```python
from build123d import *

# Parameters (mm, degrees)
EXTRUDE_1_DEPTH   = 2
HOLE_WIZARD_M81_D = 9
CHAMFER_1_SIZE    = 2


with BuildPart() as part:
    # Эскиз1 → Бобышка-Вытянуть1 (new body)
    with BuildSketch(Plane(origin=(0, 0, 0), x_dir=(1, 0, 0), z_dir=(0, 0, -1))):
        Polygon((0, 0), (0, 100), (100, 100), (100, 50), (50, 0), align=None)
    extrude(amount=EXTRUDE_1_DEPTH)

    # Отверстие с зазором M81 (through all)
    with Locations(Plane(origin=(0, 0, -2), x_dir=(1, 0, 0), z_dir=(0, 0, -1))):
        with Locations((25, 75), (25, 25), (75, 75)):
            Hole(HOLE_WIZARD_M81_D / 2)

    # Фаска1
    chamfer_1_edges = [part.edges().sort_by_distance(p)[0] for p in [
        (0, 0, -1),
        (0, -100, -1),
        (100, -100, -1),
    ]]
    chamfer(chamfer_1_edges, length=CHAMFER_1_SIZE)


solid = part.part
```
CAD build for the part. Positions are in the model's coordinates, mm. Round coordinates to 2 decimals unless told otherwise and drop trailing zeros. Order: outer loops, then holes, each group sorted by start corner. A loop starts at its lowest first (then second) coordinate and runs counter-clockwise, first axis right, second up. Notation, with made-up numbers: (-3, 82) - (45, 82) arc R9 ccw to (45, 95) - close; hole circle Ø10 at (33, 20.5). An arc over 180 degrees is marked (long way). Use CSV: the item, a comma, the result in double quotes. Start each with the question number.
1) Saw through at A-A (y = -75). List the corners of the cut face in (x, z).
2) Saw through at D-D (z = -1.2). List the corners of the cut face in (x, y), and give its area (3 significant figures).
3) Wall check: L1, parallel to X at y = -75, z = -0.6; L2, parallel to Y at x = 26, z = -1.35; L3, parallel to Y at x = 75, z = -0.5. Give the ranges that are in metal, low to high. Write a range as [from, to].
4) Saw through at B-B (x = 75). List the corners of the cut face in (y, z), and give its area (3 significant figures).
5) Saw through at C-C (y = -25). List the corners of the cut face in (x, z), and give its area (3 significant figures).
6) Two-plate mould, pull along X, no slides. Class faces 1 (the flat face through (51, -51, 0)), 2 (the flat face through (75, -25, -1)), 3 (the cylindrical face through (28.32, -28.04, -0.99)): pulls with the +X half, pulls with the -X half, needs draft (parallel to the pull), parting line crosses it, or undercut.
Values follow:
1,outline,"(0, -2) - (20.5, -2) - (20.5, 0) - (0, 0) - close; (29.5, -2) - (70.5, -2) - (70.5, 0) - (29.5, 0) - close; (79.5, -2) - (100, -2) - (100, 0) - (79.5, 0) - close"
2,outline,"(0, -98) - (2, -100) - (98, -100) - (100, -98) - (100, -50) - (50, 0) - (2, 0) - (0, -2) - close; hole circle Ø9 at (25, -75); hole circle Ø9 at (25, -25); hole circle Ø9 at (75, -75)"
2,area,"8,550 mm2"
3,L1,"x = [0, 20.5], [29.5, 70.5], [79.5, 100]"
3,L2,"y = [-100, -79.39], [-70.61, -29.39], [-20.61, 0]"
3,L3,"y = [-100, -79.5], [-70.5, -25]"
4,outline,"(-100, -2) - (-79.5, -2) - (-79.5, 0) - (-100, 0) - close; (-70.5, -2) - (-25, -2) - (-25, 0) - (-70.5, 0) - close"
4,area,"132 mm2"
5,outline,"(0, -2) - (20.5, -2) - (20.5, 0) - (0, 0) - close; (29.5, -2) - (75, -2) - (75, 0) - (29.5, 0) - close"
5,area,"132 mm2"
6,face 1,"needs draft"
6,face 2,"pulls with the +X half"
6,face 3,"undercut"
